from build123d import *

# Parameters (mm, degrees)
SKETCH1_W           = 20.701
SKETCH1_H           = 15.875
BOSS_EXTRUDE1_DEPTH = 16.51
SKETCH2_R           = 0.4191
BOSS_EXTRUDE2_DEPTH = 6.35
SKETCH3_W           = 7.874
SKETCH3_H           = 8.382
CUT_EXTRUDE1_DEPTH  = 26.134211252


with BuildPart() as part:
    # Sketch1 → Boss-Extrude1 (new body)
    with BuildSketch(Plane(origin=(0, 0, 0), x_dir=(1, 0, 0), z_dir=(0, 1, 0))):
        Rectangle(SKETCH1_W, SKETCH1_H)
    extrude(amount=BOSS_EXTRUDE1_DEPTH)

    # Sketch2 → Boss-Extrude2 (add)
    with BuildSketch(Plane(origin=(0, 0, 0), x_dir=(-1, 0, 0), z_dir=(0, -1, 0))):
        with Locations(Location((-4.7625, 0, 0), (0, 0, 90))):
            Circle(SKETCH2_R)
        with Locations(Location((4.7625, 0, 0), (0, 0, 90))):
            Circle(SKETCH2_R)
    extrude(amount=BOSS_EXTRUDE2_DEPTH)

    # Sketch3 → Cut-Extrude1 (cut, through all)
    with BuildSketch(Plane(origin=(0, 0, -7.9375), x_dir=(-1, 0, 0), z_dir=(0, 0, -1))):
        with Locations((-4.7625, 12.319)):
            Rectangle(SKETCH3_W, SKETCH3_H)
        with Locations((4.7625, 12.319)):
            Rectangle(SKETCH3_W, SKETCH3_H)
    extrude(amount=-CUT_EXTRUDE1_DEPTH, mode=Mode.SUBTRACT)


solid = part.part
The listing builds one solid part. Answer for the finished solid, in the listing's coordinates (mm). A direction names the side the tool comes from. Coordinates: 2 decimals unless noted, no trailing zeros. Order: outer loops, then holes, each group sorted by start corner. A loop starts at its lowest first (then second) coordinate and runs counter-clockwise, first axis right, second up. Notation, with made-up numbers: M 37,88 L 60,88 A9 ccw 60,94 Z; hole C 29,-6.75 d2. An arc over 180 degrees is marked long. Use CSV: the item, a comma, the result in double quotes.
Q1. Section A-A (z = 0.75) is taken. Determine the outline of the cut face in (x, y).
Here are the results:
outline,"M -10.35,0 L 10.35,0 L 10.35,16.51 L 8.7,16.51 L 8.7,8.13 L 0.83,8.13 L 0.83,16.51 L -0.83,16.51 L -0.83,8.13 L -8.7,8.13 L -8.7,16.51 L -10.35,16.51 Z"
Q2. Section D-D (x = 2.5) is taken. Determine the outline of the cut face in (y, z), then the cut area to 3 significant figures.
Here are the results:
outline,"M 0,-7.94 L 8.13,-7.94 L 8.13,7.94 L 0,7.94 Z"
area,"129 mm2"
Q3. Given pin 1 Ø8 at (x, y) = (3, -3.5) entering from +Z; pin 2 Ø3 at (x, z) = (-5.5, -0.5) entering from +Y; pin 3 Ø1.5 at (x, y) = (6, -2.5) entering from +Z; pin 4 Ø5 at (x, z) = (1.5, -3.5) entering from -Y, each flat-ended and moving along its own axis, determine where each tip first touches the part or whether it passes through.
Here are the results:
pin 1,"z = 7.94"
pin 2,"y = 8.13"
pin 3,"through"
pin 4,"y = 0"
Q4. Straight lines are drawn through the part: L1, parallel to X at y = 14.25, z = 6.5; L2, parallel to Y at x = 7, z = 6; L3, parallel to Y at x = 9.25, z = -6. For each, find the intervals that lie inside material, in ascending order.
Here are the results:
L1,"-10.35 to -8.7, -0.83 to 0.83, 8.7 to 10.35"
L2,"0 to 8.13"
L3,"0 to 16.51"
Q5. Determine the mould class of faces 1 (the cylindrical face through (4.39, -3.13, -0.19)), 2 (the flat face through (-5, -6.35, 0)), 3 (the flat face through (-10.35, 8, 0)) for opening direction X: pulls with the +X half, pulls with the -X half, needs draft (parallel to the pull), parting line crosses it, or undercut.
Here are the results:
face 1,"undercut"
face 2,"needs draft"
face 3,"pulls with the -X half"
Q6. A tool of negligible diameter and unlimited length cuts with its end or side. For faces 4 (the flat face through (-8.7, 12, 0)), 5 (the flat face through (0, 16.51, 0)), 6 (the cylindrical face through (-5.134, -3.131, -0.193)), from which of +Z, -Z, +X, -X, +Y, -Y can it reach the whole face along a straight path? Write none if from no direction.
Here are the results:
face 4,"+Z, -Z, +Y"
face 5,"+Z, -Z, +X, -X, +Y"
face 6,"-Y"
Q7. Section B-B (x = -0.5) is taken. Determine the outline of the cut face in (y, z), then the cut area to 3 significant figures.
Here are the results:
outline,"M 0,-7.94 L 16.51,-7.94 L 16.51,7.94 L 0,7.94 Z"
area,"262 mm2"
Q8. Section C-C (y = -3) is taken. Determine the outline of the cut face in (x, z), then the cut area to 3 significant figures.
Here are the results:
outline,"C -4.76,0 d0.84; C 4.76,0 d0.84"
area,"1.10 mm2"
